from build123d import *

# Parameters (mm, degrees)
F1_DEPTH = 10.922
F3_DEPTH = 33.528
F5_DEPTH = 25.4
F7_DEPTH = 25.4


# Not quite as in the source:
# - a feature names something its author has since deleted; it is built from what else it names


with BuildPart() as f1:
    # F0 (on Front) → F1 (new body)
    with BuildSketch(Plane.XZ):
        Polygon((0, 50.8), (0, 0), (63.5, 0), (63.5, 10.922), (10.922, 10.922), (10.922, 50.8), align=None)
    extrude(amount=F1_DEPTH)

    # F2 (on face) → F3 (join)
    with BuildSketch(Plane.XZ.offset(10.922)):
        Polygon((0, 10.922), (0, 0), (10.922, 0), (63.5, 0), (63.5, 10.922), (10.922, 10.922), (10.922, 50.8), (0, 50.8), align=None)
    extrude(amount=F3_DEPTH)

    # F4 (on face) → F5 (cut)
    with BuildSketch(Plane.XY.offset(10.922)):
        Polygon((63.5, -10.922), (10.922, -44.45), (63.5, -44.45), align=None)
    extrude(amount=-F5_DEPTH, mode=Mode.SUBTRACT)

    # F6 (on face) → F7 (cut)
    with BuildSketch(Plane(origin=(0, 0, 0), x_dir=(0, -1, 0), z_dir=(-1, 0, 0))):
        Polygon((27.8788925737, 50.8), (44.45, 22.098), (44.45, 50.8), align=None)
    extrude(amount=-F7_DEPTH, mode=Mode.SUBTRACT)


solid = f1.part
Design review of the part built by this model. Coordinates are the model's own, in mm. A direction names the side the tool comes from. Coordinates: 2 decimals unless noted, no trailing zeros. Order: outer loops, then holes, each group sorted by start corner. A loop starts at its lowest first (then second) coordinate and runs counter-clockwise, first axis right, second up.
Item 1: Take a section at D-D, the plane y = -36. Write out the cut boundary in (x, z).
Item 2: Take a section at C-C, the plane y = -20.5. Write out the cut boundary in (x, z), then the cut area to 3 significant figures.
Item 3: Take a section at B-B, the plane z = 8. Write out the cut boundary in (x, y), then the cut area to 3 significant figures.
Item 4: For faces 1 (the flat face through (32, -17, 10.922)), 2 (the flat face through (37.58, -27.45, 5.54)), list the 3-axis set-ups (+Z, -Z, +X, -X, +Y, -Y) from which the entire face can be reached by the end or side of a thin tool; tool diameter is ignored.
Item 5: Take a section at A-A, the plane x = 5.5. Write out the cut boundary in (y, z), then the cut area to 3 significant figures.
Item 6: For line 1 (Z direction, x = 14, y = -21); line 2 (X direction, y = -31.5, z = 5), list the stretches that pass through material, from the lowest coordinate up.
Item 7: For pin 1 Ø5 at (y, z) = (-14.5, 41.5) entering from +X; pin 2 Ø10 at (x, z) = (55.5, 20.5) entering from -Y, all flat-tipped, find the tip position at first contact; note any pin that passes through.
The answers:
1. outline: (0, 0) - (24.17, 0) - (24.17, 10.92) - (10.92, 10.92) - (10.92, 36.73) - (0, 36.73) - close
2. outline: (0, 0) - (48.48, 0) - (48.48, 10.92) - (10.92, 10.92) - (10.92, 50.8) - (0, 50.8) - close
2. area: 965 mm2
3. outline: (0, -44.45) - (10.92, -44.45) - (63.5, -10.92) - (63.5, 0) - (0, 0) - close
3. area: 1,940 mm2
4. face 1: +Z, +X, +Y, -Y
4. face 2: +Z, -Z, +X, -Y
5. outline: (-44.45, 0) - (0, 0) - (0, 50.8) - (-27.88, 50.8) - (-44.45, 22.1) - close
5. area: 2,020 mm2
6. line 1: z = 0 to 10.92
6. line 2: x = 0 to 31.23
7. pin 1: stops at x = 10.92
7. pin 2: passes through
